```python
from build123d import *

# Parameters (mm, degrees)
SCHIZZO2_W                   = 80
SCHIZZO2_H                   = 30
ESTRUSIONE_ESTRUSIONE1_DEPTH = 12.1
SCHIZZO3_R                   = 4.25
TAGLIO_ESTRUSIONE1_DEPTH     = 52.443269725
SCHIZZO4_R                   = 11.25
TAGLIO_ESTRUSIONE2_DEPTH     = 8
SCHIZZO5_R                   = 8
TAGLIO_ESTRUSIONE3_DEPTH     = 46.688510591
ESTRUSIONE_ESTRUSIONE2_START = -15
SCHIZZO6_W                   = 80
SCHIZZO6_H                   = 24.2
SCHIZZO6_R                   = 4.25
ESTRUSIONE_ESTRUSIONE2_DEPTH = 15
TAGLIO_ESTRUSIONE4_DEPTH     = 87.292583691
TAGLIO_ESTRUSIONE5_DEPTH     = 62.411806682
SCHIZZO8_R                   = 4.1
TAGLIO_ESTRUSIONE6_DEPTH     = 12
SCHIZZO10_W                  = 10.2
SCHIZZO10_H                  = 27.75
TAGLIO_ESTRUSIONE7_DEPTH     = 10.9
TAGLIO_ESTRUSIONE8_DEPTH     = 12
SCHIZZO12_W                  = 3
SCHIZZO12_H                  = 6
TAGLIO_ESTRUSIONE9_DEPTH     = 8.2


with BuildPart() as part:
    # Schizzo2 → Estrusione-Estrusione1 (new, symmetric)
    with BuildSketch(Plane.XY):
        Rectangle(SCHIZZO2_W, SCHIZZO2_H)
    extrude(amount=ESTRUSIONE_ESTRUSIONE1_DEPTH, both=True)

    # Schizzo3 → Taglio-Estrusione1 (cut, through all)
    with BuildSketch(Plane.XZ.offset(15)):
        with Locations(Location((32.5, -4.6, 0), (0, 0, 270))):
            Circle(SCHIZZO3_R)
    extrude(amount=-TAGLIO_ESTRUSIONE1_DEPTH, mode=Mode.SUBTRACT)

    # Schizzo4 → Taglio-Estrusione2 (cut)
    with BuildSketch(Plane.XY.offset(12.1)):
        with Locations((0.9, 0)):
            Circle(SCHIZZO4_R)
    extrude(amount=-TAGLIO_ESTRUSIONE2_DEPTH, mode=Mode.SUBTRACT)

    # Schizzo5 → Taglio-Estrusione3 (cut, through all)
    with BuildSketch(Plane.XY.offset(4.1)):
        with Locations((0.9, 0)):
            Circle(SCHIZZO5_R)
    extrude(amount=-TAGLIO_ESTRUSIONE3_DEPTH, mode=Mode.SUBTRACT)

    # Schizzo6 → Estrusione-Estrusione2 (add)
    with BuildSketch(Plane(origin=(0, -15, 0), x_dir=(1, 0, 0), z_dir=(0, 1, 0)).offset(ESTRUSIONE_ESTRUSIONE2_START)):
        Rectangle(SCHIZZO6_W, SCHIZZO6_H)
        with Locations(Location((32.5, 4.6, 0), (0, 0, 90))):
            Circle(SCHIZZO6_R, mode=Mode.SUBTRACT)
    extrude(amount=ESTRUSIONE_ESTRUSIONE2_DEPTH)

    # Schizzo7 → Taglio-Estrusione4 (cut, through all)
    with BuildSketch(Plane(origin=(40, 0, 0), x_dir=(0, 0, -1), z_dir=(1, 0, 0))):
        with BuildLine():
            Line((-2.146261356, -18.25), (-7.053738644, -18.25))
            Line((-7.053738644, -18.25), (-8.280607966, -20.375))
            ThreePointArc((-8.280607966, -20.375), (-4.6, -26.75), (-0.919392034, -20.375))
            Line((-0.919392034, -20.375), (-2.146261356, -18.25))
        make_face()
    extrude(amount=-TAGLIO_ESTRUSIONE4_DEPTH, mode=Mode.SUBTRACT)

    # Schizzo9 → Taglio-Estrusione5 (cut, through all)
    with BuildSketch(Plane.XZ.offset(-15)):
        Polygon((25, -12.1), (19.688377523, -2.9), (-40, -2.9), (-40, -12.1), align=None)
    extrude(amount=TAGLIO_ESTRUSIONE5_DEPTH, mode=Mode.SUBTRACT)

    # Schizzo8 → Taglio-Estrusione6 (cut)
    with BuildSketch(Plane.XY.offset(12.1)):
        with Locations((-29.1, 0)):
            Circle(SCHIZZO8_R)
    extrude(amount=-TAGLIO_ESTRUSIONE6_DEPTH, mode=Mode.SUBTRACT)

    # Schizzo10 → Taglio-Estrusione7 (cut)
    with BuildSketch(Plane.ZY.offset(40)):
        with Locations((7, 1.125)):
            Rectangle(SCHIZZO10_W, SCHIZZO10_H)
    extrude(amount=-TAGLIO_ESTRUSIONE7_DEPTH, mode=Mode.SUBTRACT)

    # Schizzo11 → Taglio-Estrusione8 (cut)
    with BuildSketch(Plane.ZY.offset(29.1)):
        with BuildLine():
            Line((8.110362971, 6.25), (6.089637029, 6.25))
            Line((6.089637029, 6.25), (5.584455543, 7.125))
            ThreePointArc((5.584455543, 7.125), (7.1, 9.75), (8.615544457, 7.125))
            Line((8.615544457, 7.125), (8.110362971, 6.25))
        make_face()
        with BuildLine():
            Line((8.110362971, -9.75), (6.089637029, -9.75))
            Line((6.089637029, -9.75), (5.584455543, -8.875))
            ThreePointArc((5.584455543, -8.875), (7.1, -6.25), (8.615544457, -8.875))
            Line((8.615544457, -8.875), (8.110362971, -9.75))
        make_face()
    extrude(amount=-TAGLIO_ESTRUSIONE8_DEPTH, mode=Mode.SUBTRACT)

    # Schizzo12 → Taglio-Estrusione9 (cut)
    with BuildSketch(Plane.XY.offset(12.1)):
        with Locations((-21.6, -8)):
            Rectangle(SCHIZZO12_W, SCHIZZO12_H)
        with Locations((-21.6, 8)):
            Rectangle(SCHIZZO12_W, SCHIZZO12_H)
    extrude(amount=-TAGLIO_ESTRUSIONE9_DEPTH, mode=Mode.SUBTRACT)


solid = part.part
```
The model under review builds one solid part; all positions refer to its coordinate system, in mm. A direction names the side the tool comes from. Round coordinates to 2 decimals unless told otherwise and drop trailing zeros. Order: outer loops, then holes, each group sorted by start corner. A loop starts at its lowest first (then second) coordinate and runs counter-clockwise, first axis right, second up.
Item 1: Machinability: for faces 1 (the flat face through (-20.1, -7, 9)), 2 (the flat face through (40, -8, 0)), 3 (the flat face through (-29.1, 11, 7)), 4 (the flat face through (-19, 6.25, 7)), which of the approach directions +Z, -Z, +X, -X, +Y, -Y give a long, thin tool a straight path to every point of the face, cutting with its end or side? Answer none if there is none.
Working result:
face 1: +Z
face 2: +Z, -Z, +X, +Y, -Y
face 3: +Z, -X, +Y
face 4: -X
Item 2: Add section D-D, the plane x = -21. State the section outline as (y, z) points (3 decimals).
Working result:
outline: (-30, -2.9) - (15, -2.9) - (15, 12.1) - (11, 12.1) - (11, 3.9) - (5, 3.9) - (5, 12.1) - (-5, 12.1) - (-5, 3.9) - (-11, 3.9) - (-11, 12.1) - (-30, 12.1) - close; hole (-20.375, 0.919) - (-18.25, 2.146) - (-18.25, 7.054) - (-20.375, 8.281) arc R4.25 ccw (long way) to start
Item 3: Draft analysis for pull direction Z (two halves, no side actions). For faces 5 (the flat face through (-20.1, 9, 9)), 6 (the cylindrical face through (-18.62, -6.25, 7.05)), 7 (the flat face through (-10, -7, -2.9)), state which applies: released by +Z, released by -Z, zero draft, split by the parting line, or undercut.
Working result:
face 5: zero draft
face 6: undercut
face 7: released by -Z
Item 4: Add section C-C, the plane z = -2. State the section outline as (x, y) points, and give its area (3 significant figures).
Working result:
outline: (-40, -30) - (29.14, -30) - (29.14, 15) - (-40, 15) - close; (35.86, -30) - (40, -30) - (40, 15) - (35.86, 15) - close; hole circle Ø16 at (0.9, 0)
area: 3,100 mm2
Item 5: Add section B-B, the plane y = -22.5. State the section outline as (x, z) points.
Working result:
outline: (-40, -2.9) - (19.69, -2.9) - (25, -12.1) - (40, -12.1) - (40, 0.35) - (-40, 0.35) - close; (-40, 8.85) - (40, 8.85) - (40, 12.1) - (-40, 12.1) - close; hole circle Ø8.5 at (32.5, -4.6)
Item 6: To check wall thickness, follow probe 1 along Z at (x, y) = (-26.1, -8); probe 2 along Y at (x, z) = (-24.5, 7); probe 3 along Y at (x, z) = (-6.5, 4.5). State the ranges of each line that lie inside material, in increasing order.
Working result:
probe 1: z = -2.9 to 5.35, 8.85 to 12.1
probe 2: y = -30 to -26.01, -18.25 to -9.75, -6.25 to 6.25, 9.75 to 15
probe 3: y = -30 to -26.75, -18.25 to -8.47, 8.47 to 15
Item 7: Add section A-A, the plane x = 0.9. State the section outline as (y, z) points (3 decimals), and give its area (3 significant figures).
Working result:
outline: (-30, -2.9) - (-8, -2.9) - (-8, 4.1) - (-11.25, 4.1) - (-11.25, 12.1) - (-30, 12.1) - close; (8, -2.9) - (15, -2.9) - (15, 12.1) - (11.25, 12.1) - (11.25, 4.1) - (8, 4.1) - close; hole (-20.375, 0.919) - (-18.25, 2.146) - (-18.25, 7.054) - (-20.375, 8.281) arc R4.25 ccw (long way) to start
area: 324 mm2
Item 8: For pin 1 (6 mm diameter, centred on x = -14, y = -16, fed in from -Z); pin 2 (2.5 mm diameter, centred on x = -31, y = -1, fed in from +Z); pin 3 (1.8 mm diameter, centred on y = -7.5, z = 7, fed in from -X), all flat-tipped, find the tip position at first contact; note any pin that passes through.
Working result:
pin 1: stops at z = -2.9
pin 2: stops at z = 0.1
pin 3: stops at x = -17.1
